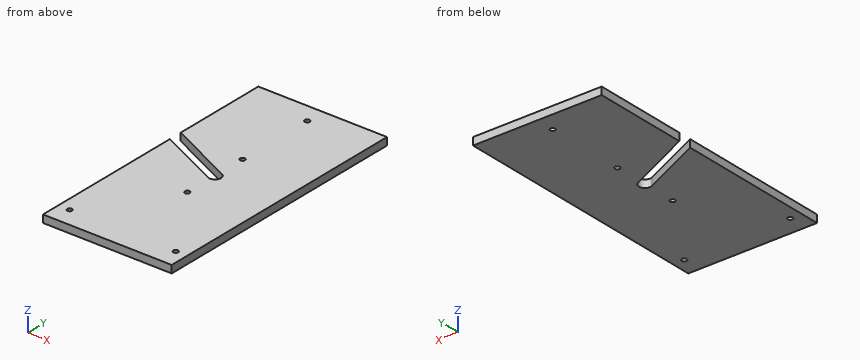
from build123d import *

# Parameters (mm, degrees)
AUFSATZ_LINEAR_AUSTRAGEN1_DEPTH  = 10
F_6_5_6_5_DURCHMESSER_BOHRUNG5_D = 6.5


with BuildPart() as part:
    # Skizze1 → Aufsatz-Linear austragen1 (new body)
    with BuildSketch(Plane.XY):
        with BuildLine():
            Line((85, 175), (-85, 175))
            Line((-85, 175), (-85, 48.841550225))
            Line((-85, 48.841550225), (3.406376291, 7.238549618))
            ThreePointArc((3.406376291, 7.238549618), (7.238549618, -3.406376291), (-3.406376291, -7.238549618))
            Line((-3.406376291, -7.238549618), (-85, 31.158449775))
            Line((-85, 31.158449775), (-85, -175))
            Line((-85, -175), (85, -175))
            Line((85, -175), (85, 175))
        make_face()
    extrude(amount=AUFSATZ_LINEAR_AUSTRAGEN1_DEPTH)

    # Ø6.5 (6.5) Durchmesser Bohrung5 (through all)
    with Locations(Plane.XY.offset(10)):
        with Locations((0, 150), (-70, -150), (70, -150), (0, 45), (0, -45)):
            Hole(F_6_5_6_5_DURCHMESSER_BOHRUNG5_D / 2)


solid = part.part
Could you check a few things on this model? Use its own coordinates, in mm. Give positions to 0.01 mm unless a question says otherwise; leave off trailing zeros. Write each loop counter-clockwise with the first axis right and the second up, starting at its lowest first coordinate (ties: lowest second). Pieces come first, ordered by that corner, then holes. Notation, with made-up numbers: (57.25, 20) -> (87.25, 20) arc R9 cw to (87.25, 28) -> close; hole circle Ø10 at (-16, 43.5). An arc over 180 degrees is marked (long way). Answer as CSV lines item,"result". Start each with the question number.
(1) If we section it at B-B, the plane y = -150: Write out the boundary of the cut face in (x, z), and give its area (3 significant figures).
(2) If we section it at C-C, the plane y = 0: Write out the boundary of the cut face in (x, z), and give its area (3 significant figures).
(3) I'm going to push a flat-ended pin straight in: pin 1 Ø4 at (x, y) = (70, -150) entering from +Z. Where does the tip first touch, or does it pass through?
(4) If we section it at A-A, the plane x = 70: Write out the boundary of the cut face in (y, z).
(5) Please list where these lines run through material, in increasing order: line 1 (X direction, y = -45.5, z = 8.75); line 2 (Y direction, x = 70, z = 4.25); line 3 (Y direction, x = 0, z = 4.75).
(6) If we section it at D-D, the plane z = 1.75: Write out the boundary of the cut face in (x, y), and give its area (3 significant figures).
Answer list:
1,outline,"(-85, 0) -> (-73.25, 0) -> (-73.25, 10) -> (-85, 10) -> close; (-66.75, 0) -> (66.75, 0) -> (66.75, 10) -> (-66.75, 10) -> close; (73.25, 0) -> (85, 0) -> (85, 10) -> (73.25, 10) -> close"
1,area,"1,570 mm^2"
2,outline,"(-85, 0) -> (-18.79, 0) -> (-18.79, 10) -> (-85, 10) -> close; (8, 0) -> (85, 0) -> (85, 10) -> (8, 10) -> close"
2,area,"1,430 mm^2"
3,pin 1,"through"
4,outline,"(-175, 0) -> (-153.25, 0) -> (-153.25, 10) -> (-175, 10) -> close; (-146.75, 0) -> (175, 0) -> (175, 10) -> (-146.75, 10) -> close"
5,line 1,"-85 to -3.21, 3.21 to 85"
5,line 2,"-175 to -153.25, -146.75 to 175"
5,line 3,"-175 to -48.25, -41.75 to -8, 8.84 to 41.75, 48.25 to 146.75, 153.25 to 175"
6,outline,"(-85, -175) -> (85, -175) -> (85, 175) -> (-85, 175) -> (-85, 48.84) -> (3.41, 7.24) arc R8 cw to (-3.41, -7.24) -> (-85, 31.16) -> close; hole circle Ø6.5 at (-70, -150); hole circle Ø6.5 at (0, -45); hole circle Ø6.5 at (0, 45); hole circle Ø6.5 at (0, 150); hole circle Ø6.5 at (70, -150)"
6,area,"57,700 mm^2"
